from build123d import *
from build123d.topology import SkipClean

# Parameters (mm, degrees)
SKETCH_1_R      = 1.5
EXTRUDE_1_DEPTH = 3
SKETCH_2_W      = 23.5
SKETCH_2_H      = 11
SKETCH_2_R      = 1.5
SKETCH_2_W_2    = 0.1
SKETCH_2_W_3    = 15
EXTRUDE_2_DEPTH = 7
EXTRUDE_3_DEPTH = 8
FILLET_4_R      = 3
EXTRUDE_4_DEPTH = 23.6
FILLET_5_R      = 5
FILLET_6_R      = 3
EXTRUDE_START   = 3
SKETCH_7_R      = 3.5
SKETCH_7_R_2    = 1.5
EXTRUDE_5_DEPTH = 3


with BuildPart() as part:
    # 草图1 → 凸台-拉伸1 (new body)
    with BuildSketch(Plane(origin=(0, 0, 0), x_dir=(1, 0, 0), z_dir=(0, 1, 0))):
        Polygon((-23.5, 19), (-23.5, -19), (0.1, -19), (0.1, -5), (14.1, -5), (14.1, -19), (23.5, -19), (23.5, 19), align=None)
        with Locations(Location((-19.5, -14, 0), (0, 0, 270))):
            Circle(SKETCH_1_R, mode=Mode.SUBTRACT)
        with Locations(Location((19.5, -14, 0), (0, 0, 270))):
            Circle(SKETCH_1_R, mode=Mode.SUBTRACT)
        with Locations(Location((-19.5, 14, 0), (0, 0, 270))):
            Circle(SKETCH_1_R, mode=Mode.SUBTRACT)
        with Locations(Location((19.5, 14, 0), (0, 0, 270))):
            Circle(SKETCH_1_R, mode=Mode.SUBTRACT)
    extrude(amount=EXTRUDE_1_DEPTH)

    # 草图2 → 凸台-拉伸2 (add)
    # profile 1 of 3: a face of its own
    with BuildSketch(Plane.XY.offset(19)):
        with Locations((-11.75, 5.5)):
            Rectangle(SKETCH_2_W, SKETCH_2_H)
        with Locations((-20, 7)):
            Circle(SKETCH_2_R, mode=Mode.SUBTRACT)
        with Locations((-12, 7)):
            Circle(SKETCH_2_R, mode=Mode.SUBTRACT)
    # profile 2 of 3: a face of its own
    with BuildSketch(Plane.XY.offset(19)):
        with Locations((0.05, 5.5)):
            Rectangle(SKETCH_2_W_2, SKETCH_2_H)
    # profile 3 of 3: a face of its own
    with BuildSketch(Plane.XY.offset(19)):
        with Locations((16, 5.5)):
            Rectangle(SKETCH_2_W_3, SKETCH_2_H)
        with Locations((12, 7)):
            Circle(SKETCH_2_R, mode=Mode.SUBTRACT)
        with Locations((20, 7)):
            Circle(SKETCH_2_R, mode=Mode.SUBTRACT)
    extrude(amount=EXTRUDE_2_DEPTH)

    # 草图3 → 凸台-拉伸3 (add)
    with BuildSketch(Plane(origin=(0.1, 0, 0), x_dir=(0, 0, -1), z_dir=(1, 0, 0))):
        Polygon((-19, 11), (-19, 8), (-4, 3), (5, 3), align=None)
    extrude(amount=-EXTRUDE_3_DEPTH)

    # 圆角4
    fillet_4_edges = [part.edges().sort_by_distance(p)[0] for p in [
        (-23.5, 11, 22.5),
        (23.5, 11, 22.5),
        (8.5, 11, 22.5),
    ]]
    fillet(fillet_4_edges, radius=FILLET_4_R)

    # 草图4 → 凸台-拉伸4 (add)
    with BuildSketch(Plane.ZY.offset(23.5)):
        Polygon((26, 0), (26, -5), (23, -5), (19.5, 0), align=None)
    extrude(amount=-EXTRUDE_4_DEPTH)

    # 圆角5
    fillet_5_edges = [part.edges().sort_by_distance(p)[0] for p in [
        (14.1, 1.5, 19),
    ]]
    fillet(fillet_5_edges, radius=FILLET_5_R)

    # 圆角6
    fillet_6_edges = [part.edges().sort_by_distance(p)[0] for p in [
        (-23.5, 1.5, -19),
        (23.5, 1.5, -19),
    ]]
    fillet(fillet_6_edges, radius=FILLET_6_R)

    # 草图7 → 凸台-拉伸5 (add)
    with SkipClean():  # the faces are left unmerged after this step: merging them gives an invalid solid
        with BuildSketch(Plane(origin=(0, 0, 19), x_dir=(-1, 0, 0), z_dir=(0, 0, -1)).offset(EXTRUDE_START)):
            with Locations(Location((12, 7, 0), (0, 0, 180))):
                Circle(SKETCH_7_R)
            with Locations((12, 7)):
                Circle(SKETCH_7_R_2, mode=Mode.SUBTRACT)
        extrude(amount=-EXTRUDE_5_DEPTH)


solid = part.part
Work out the finished part from the listing and answer in its coordinate system (mm). A direction names the side the tool comes from. Round coordinates to 2 decimals unless told otherwise and drop trailing zeros. Order: outer loops, then holes, each group sorted by start corner. A loop starts at its lowest first (then second) coordinate and runs counter-clockwise, first axis right, second up. Notation, with made-up numbers: M 88.25,29.5 L 96.25,29.5 A28 ccw 96.25,54.5 Z; hole C 24.5,-22 d3. An arc over 180 degrees is marked long. One line per item, written item: value.
Q1. Determine the mould class of faces 6 (the face through (12.67, 1.52, 17.5)), 7 (the face through (-10, 11, 22)), 8 (the face through (-22.64, 10.1, 22.55)) for opening direction X: released by +X, released by -X, zero draft, split by the parting line, or undercut.
Derived:
face 6: undercut
face 7: zero draft
face 8: released by -X
Q2. Flat-ended cylindrical pins translate along their axes: pin 1 (10 mm diameter, centred on x = -12, z = 11.5, fed in from -Y); pin 2 (1 mm diameter, centred on y = 5, z = 1.5, fed in from +X); pin 3 (3.5 mm diameter, centred on x = -20, y = 7, fed in from -Z). Find the tip coordinate at first contact, or state that the pin passes through.
Derived:
pin 1: y = 0
pin 2: x = 0.1
pin 3: z = 19
Q3. For faces 1 (the face through (0.1, 1, 18)), 2 (the face through (11.675, 5.536, 22.451)), 3 (the face through (14.1, 1, 9)), 4 (the face through (-14.8, 9.1, 17.5)), 5 (the face through (16, 11, 22)), determine the directions among +Z, -Z, +X, -X, +Y, -Y from which every point of the face is accessible in a straight line to the end or side of a thin tool.
Derived:
face 1: +Z, +Y
face 2: +Z, -Z
face 3: +Y, -Y
face 4: -Z
face 5: +Z, -Z, +X, -X, +Y
Q4. Straight lines are drawn through the part: line 1 (X direction, y = 1.9, z = -14); line 2 (X direction, y = 1.6, z = 14); line 3 (Y direction, x = 12, z = 22.5). For each, find the intervals that lie inside material, in ascending order.
Derived:
line 1: -23.5 to -21, -18 to 18, 21 to 23.5
line 2: -23.5 to -21, -18 to 0.1, 14.1 to 18, 21 to 23.5
line 3: 0 to 5.5, 8.5 to 11
Q5. Find section B-B on y = 0.75. Write down the section's boundary in (x, z).
Derived:
outline: M -23.5,-16 A3 ccw -20.5,-19 L 20.5,-19 A3 ccw 23.5,-16 L 23.5,26 L 8.5,26 L 8.5,19 L 9.1,19 A5 cw 14.1,14 L 14.1,5 L 0.1,5 L 0.1,26 L -23.5,26 Z; hole C -19.5,-14 d3; hole C -19.5,14 d3; hole C 19.5,-14 d3; hole C 19.5,14 d3
Q6. Find section D-D on x = -19.5. Write down the section's boundary in (y, z).
Derived:
outline: M -5,23 L 0,19.5 L 0,15.5 L 3,15.5 L 3,19 L 5.59,19 L 5.59,26 L -5,26 Z; M 0,-19 L 3,-19 L 3,-15.5 L 0,-15.5 Z; M 0,-12.5 L 3,-12.5 L 3,12.5 L 0,12.5 Z; M 8.41,19 L 11,19 L 11,26 L 8.41,26 Z
Q7. Find section A-A on z = -14. Write down the section's boundary in (x, y), then the cut area to 3 significant figures.
Derived:
outline: M -23.5,0 L -21,0 L -21,3 L -23.5,3 Z; M -18,0 L 18,0 L 18,3 L -18,3 Z; M 21,0 L 23.5,0 L 23.5,3 L 21,3 Z
area: 123 mm²
